```python
from build123d import *

# Parameters (mm, degrees)
SKETCH1_W           = 50
SKETCH1_H           = 90
BOSS_EXTRUDE1_DEPTH = 0.889
SKETCH2_R           = 2.75
CUT_EXTRUDE1_DEPTH  = 117.345408204
BREAK_CORNER1_DEPTH = 0.889
EDGE_FLANGE1_DEPTH  = 80
BREAK_CORNER2_START = 49.812591379
BREAK_CORNER2_DEPTH = 0.889


# Read off the part's stored shape, not the designer's step: Break-Corner1, Break-Corner2
# Sheet-metal steps are written as plain solids
with BuildPart() as part:
    # Sketch1 → Boss-Extrude1 (new body)
    with BuildSketch(Plane.XY):
        with Locations((76.701591379, -11.5)):
            Rectangle(SKETCH1_W, SKETCH1_H)
    extrude(amount=BOSS_EXTRUDE1_DEPTH)

    # Sketch2 → Cut-Extrude1 (cut, through all)
    with BuildSketch(Plane(origin=(0, 0, 0.889), x_dir=(-1, 0, 0), z_dir=(0, 0, -1))):
        with Locations((-61.701591379, -41.5)):
            Circle(SKETCH2_R)
        with Locations((-91.701591379, -41.5)):
            Circle(SKETCH2_R)
        with BuildLine():
            Line((-64.001591379, -21.5), (-64.001591379, 18.5))
            ThreePointArc((-64.001591379, 18.5), (-61.701591379, 20.8), (-59.401591379, 18.5))
            Line((-59.401591379, 18.5), (-59.401591379, -21.5))
            ThreePointArc((-59.401591379, -21.5), (-61.701591379, -23.8), (-64.001591379, -21.5))
        make_face()
        with BuildLine():
            Line((-94.001591379, -21.5), (-94.001591379, 18.5))
            ThreePointArc((-94.001591379, 18.5), (-91.701591379, 20.8), (-89.401591379, 18.5))
            Line((-89.401591379, 18.5), (-89.401591379, -21.5))
            ThreePointArc((-89.401591379, -21.5), (-91.701591379, -23.8), (-94.001591379, -21.5))
        make_face()
    extrude(amount=CUT_EXTRUDE1_DEPTH, mode=Mode.SUBTRACT)

    # Break-Corner1 outline → Break-Corner1 (cut)
    with BuildSketch(Plane.XY):
        with BuildLine():
            ThreePointArc((51.701591379, 28.5), (53.166057473, 32.035533906), (56.701591379, 33.5))
            Line((56.701591379, 33.5), (51.701591379, 33.5))
            Line((51.701591379, 33.5), (51.701591379, 28.5))
        make_face()
        with BuildLine():
            Line((101.701591379, 33.5), (96.701591379, 33.5))
            ThreePointArc((96.701591379, 33.5), (100.237125285, 32.035533906), (101.701591379, 28.5))
            Line((101.701591379, 28.5), (101.701591379, 33.5))
        make_face()
        with BuildLine():
            ThreePointArc((56.701591379, -56.5), (53.166057474, -55.035533906), (51.701591379, -51.5))
            Line((51.701591379, -51.5), (51.701591379, -56.5))
            Line((51.701591379, -56.5), (56.701591379, -56.5))
        make_face()
        with BuildLine():
            Line((101.701591379, -56.5), (101.701591379, -51.5))
            ThreePointArc((101.701591379, -51.5), (100.237125285, -55.035533906), (96.701591379, -56.5))
            Line((96.701591379, -56.5), (101.701591379, -56.5))
        make_face()
    extrude(amount=BREAK_CORNER1_DEPTH, mode=Mode.SUBTRACT)

    # Edge-Flange1 section (across the edge) → Edge-Flange1 (add)
    with BuildSketch(Plane(origin=(50.701591379, 28.5, 0.889), x_dir=(1, 0, 0), z_dir=(0, -1, 0))):
        with BuildLine():
            Line((-0.889, 1), (-0.889, 11.811))
            Line((-0.889, 11.811), (0, 11.811))
            Line((0, 11.811), (0, 1))
            ThreePointArc((0, 1), (0.292893219, 0.292893219), (1, 0))
            Line((1, 0), (1, -0.889))
            ThreePointArc((1, -0.889), (-0.33572471, -0.33572471), (-0.889, 1))
        make_face()
    extrude(amount=EDGE_FLANGE1_DEPTH)

    # Break-Corner2 outline → Break-Corner2 (cut)
    with BuildSketch(Plane.YZ.offset(BREAK_CORNER2_START)):
        with BuildLine():
            ThreePointArc((-51.5, 2.7), (-48.571067812, 9.771067812), (-41.5, 12.7))
            Line((-41.5, 12.7), (-51.5, 12.7))
            Line((-51.5, 12.7), (-51.5, 2.7))
        make_face()
        with BuildLine():
            Line((28.5, 12.7), (18.5, 12.7))
            ThreePointArc((18.5, 12.7), (25.571067812, 9.771067812), (28.5, 2.7))
            Line((28.5, 2.7), (28.5, 12.7))
        make_face()
    extrude(amount=BREAK_CORNER2_DEPTH, mode=Mode.SUBTRACT)


solid = part.part
```
Model file for the job. Use its own axes, mm. A direction names the side the tool comes from. Coordinates: 2 decimals unless noted, no trailing zeros. Loops run counter-clockwise (first coordinate to the right, second up) from the corner with the lowest first, then second, coordinate; pieces in that order, holes last. Notation, with made-up numbers: M -24.75,57 L -4.75,57 A23 cw -4.75,84 Z; hole C 23,78.25 d10. An arc over 180 degrees is marked long. Use CSV: the item, a comma, the result in double quotes. Start each with the question number.
1. Band-saw the part on D-D, the plane x = 79.5. List the corners of the cut face in (y, z).
2. Band-saw the part on C-C, the plane z = 5.5. List the corners of the cut face in (x, y), then the cut area to 3 significant figures.
3. Flat gauge pins, fed straight in: pin 1 (1.5 mm diameter, centred on x = 51, z = 1.5, fed in from -Y); pin 2 (2 mm diameter, centred on x = 90, y = -30, fed in from +Z); pin 3 (3 mm diameter, centred on y = -5, z = 8.5, fed in from +X). Where does each tip first touch, or does it go through?
4. Probe probe 1 along X at (y, z) = (-41.5, 0.75); probe 2 along X at (y, z) = (1.5, 5); probe 3 along X at (y, z) = (-41.5, 0.65). List the from-to ranges inside material, lowest first. Write a range as [from, to].
5. Tool access for faces 1 (the flat face through (76, -11, 0.889)), 2 (the cylindrical face through (91.7, -23.8, 0.5)), 3 (the flat face through (50.6, 28.5, 1.4)): list every direction of +Z, -Z, +X, -X, +Y, -Y with a clear straight run to the whole face (end or side of a thin tool).
6. Two-plate mould, pull along X, no slides. Class faces 4 (the flat face through (50.702, -11, 7)), 5 (the cylindrical face through (61.75, 20.8, 0.45)), 6 (the flat face through (50.6, -51.5, 1.4)): pulls with the +X half, pulls with the -X half, needs draft (parallel to the pull), parting line crosses it, or undercut.
7. Band-saw the part on B-B, the plane x = 90.5. List the corners of the cut face in (y, z).
8. Band-saw the part on A-A, the plane y = -16.5. List the corners of the cut face in (x, z).
Entries:
1,outline,"M -56.5,0 L 33.5,0 L 33.5,0.89 L -56.5,0.89 Z"
2,outline,"M 49.81,-51.1 L 50.7,-51.1 L 50.7,28.1 L 49.81,28.1 Z"
2,area,"70.4 mm2"
3,pin 1,"stops at y = -51.5"
3,pin 2,"stops at z = 0.89"
3,pin 3,"stops at x = 50.7"
4,probe 1,"x = [50.19, 58.95], [64.45, 88.95], [94.45, 101.7]"
4,probe 2,"x = [49.81, 50.7]"
4,probe 3,"x = [50.28, 58.95], [64.45, 88.95], [94.45, 101.7]"
5,face 1,"+Z, +X, +Y, -Y"
5,face 2,"+Z, -Z"
5,face 3,"+Z, -Z, -X, +Y"
6,face 4,"pulls with the +X half"
6,face 5,"undercut"
6,face 6,"needs draft"
7,outline,"M -56.5,0 L -43.97,0 L -43.97,0.89 L -56.5,0.89 Z; M -39.03,0 L -23.46,0 L -23.46,0.89 L -39.03,0.89 Z; M 20.46,0 L 33.5,0 L 33.5,0.89 L 20.46,0.89 Z"
8,outline,"M 49.81,1.89 A1.89 ccw 51.7,0 L 59.4,0 L 59.4,0.89 L 51.7,0.89 A1 cw 50.7,1.89 L 50.7,12.7 L 49.81,12.7 Z; M 64,0 L 89.4,0 L 89.4,0.89 L 64,0.89 Z; M 94,0 L 101.7,0 L 101.7,0.89 L 94,0.89 Z"
